```python
from build123d import *

# Parameters (mm, degrees)
SKETCH1_W           = 58.42
SKETCH1_H           = 58.42
SKETCH1_R           = 2.1
SKETCH1_R_2         = 5.5
SKETCH1_R_3         = 2.05
BOSS_EXTRUDE1_DEPTH = 6.35
CHAMFER1_SIZE       = 2.48
CHAMFER2_SIZE       = 3.1


with BuildPart() as part:
    # Sketch1 → Boss-Extrude1 (new body)
    with BuildSketch(Plane(origin=(0, 0, 0), x_dir=(1, 0, 0), z_dir=(0, 1, 0))):
        with Locations((29.21, 29.21)):
            Rectangle(SKETCH1_W, SKETCH1_H)
        with Locations(Location((5.64, 52.78, 0), (0, 0, 270))):
            Circle(SKETCH1_R, mode=Mode.SUBTRACT)
        with Locations(Location((52.78, 52.78, 0), (0, 0, 270))):
            Circle(SKETCH1_R, mode=Mode.SUBTRACT)
        with Locations(Location((52.78, 5.64, 0), (0, 0, 270))):
            Circle(SKETCH1_R, mode=Mode.SUBTRACT)
        with Locations(Location((5.64, 5.64, 0), (0, 0, 270))):
            Circle(SKETCH1_R, mode=Mode.SUBTRACT)
        with Locations(Location((29.21, 29.21, 0), (0, 0, 270))):
            Circle(SKETCH1_R_2, mode=Mode.SUBTRACT)
        with Locations(Location((13.653650814, 44.766349186, 0), (0, 0, 270))):
            Circle(SKETCH1_R_3, mode=Mode.SUBTRACT)
        with Locations(Location((44.766349186, 44.766349186, 0), (0, 0, 270))):
            Circle(SKETCH1_R_3, mode=Mode.SUBTRACT)
        with Locations(Location((44.766349186, 13.653650814, 0), (0, 0, 270))):
            Circle(SKETCH1_R_3, mode=Mode.SUBTRACT)
        with Locations(Location((13.653650814, 13.653650814, 0), (0, 0, 270))):
            Circle(SKETCH1_R_3, mode=Mode.SUBTRACT)
    extrude(amount=BOSS_EXTRUDE1_DEPTH)

    # Chamfer1
    chamfer1_edges = [part.edges().sort_by_distance(p)[0] for p in [
        (13.653650814, 0, -46.816349186),
        (44.766349186, 0, -46.816349186),
        (44.766349186, 0, -15.703650814),
        (13.653650814, 0, -15.703650814),
    ]]
    chamfer(chamfer1_edges, length=CHAMFER1_SIZE)

    # Chamfer2
    chamfer2_edges = [part.edges().sort_by_distance(p)[0] for p in [
        (5.64, 6.35, -54.88),
        (52.78, 6.35, -54.88),
        (52.78, 6.35, -7.74),
        (5.64, 6.35, -7.74),
    ]]
    chamfer(chamfer2_edges, length=CHAMFER2_SIZE)


solid = part.part
```
Input: part model. Units: mm. Frame: model coordinates. Round coordinates to 2 decimals unless told otherwise and drop trailing zeros. Order: outer loops, then holes, each group sorted by start corner. A loop starts at its lowest first (then second) coordinate and runs counter-clockwise, first axis right, second up. Notation, with made-up numbers: (50.5, 62) - (94.5, 62) arc R8 ccw to (94.5, 74) - close; hole circle Ø11 at (68, 5.25). An arc over 180 degrees is marked (long way). One line per question, with ' | ' between items. Start each with the question number.
1) Cut plane C-C, the plane x = 29.21. Return the cut outline in (y, z).
2) Cut plane A-A, the plane x = 52.78. Return the cut outline in (y, z), then the cut area to 3 significant figures.
3) Pull-direction query (Z, two-part tool) for faces 1 (the flat face through (22, 6.35, -30)), 2 (the conical face through (6.316, 3.401, -3.493)), 3 (the flat face through (29, 3, -58.42)); classes: +Z half, -Z half, draft (parallel to the pull), parting line (faces both ways), or undercut.
4) Contact query for flat-ended pins moving along their axis: P1, Ø4.5, axis at x = 13.65, z = -44.77, coming from the -Y side; P2, Ø4, axis at x = 52.78, z = -5.64, coming from the -Y side; P3, Ø5.5, axis at x = 5.64, z = -52.78, coming from the +Y side; P4, Ø6.5, axis at x = 5.64, z = -5.64, coming from the +Y side. Output: stop coordinate, or through.
5) Cut plane D-D, the plane y = 4. Give the number of separate pieces and of enclosed holes in the cut face, then the cut area to 3 significant figures.
6) Cut plane B-B, the plane z = -5.64. Return the cut outline in (x, y), then the cut area to 3 significant figures.
7) Ray query, probe 1 along X at (y, z) = (1.15, -52.78); probe 2 along Z at (x, y) = (14, 4.5); probe 3 along X at (y, z) = (5.75, -46). Return the intervals inside material, ascending.
Worked out:
1) outline: (0, -58.42) - (6.35, -58.42) - (6.35, -34.71) - (0, -34.71) - close; (0, -23.71) - (6.35, -23.71) - (6.35, 0) - (0, 0) - close
2) outline: (0, -58.42) - (6.35, -58.42) - (6.35, -57.98) - (3.25, -54.88) - (0, -54.88) - close; (0, -50.68) - (3.25, -50.68) - (6.35, -47.58) - (6.35, -10.84) - (3.25, -7.74) - (0, -7.74) - close; (0, -3.54) - (3.25, -3.54) - (6.35, -0.44) - (6.35, 0) - (0, 0) - close | area: 298 mm^2
3) face 1: draft | face 2: undercut | face 3: -Z half
4) P1: stops at y = 2.27 | P2: passes through | P3: stops at y = 3.9 | P4: stops at y = 4.4
5) separate pieces: 1 | enclosed holes: 9 | area: 3,160 mm^2
6) outline: (0, 0) - (3.54, 0) - (3.54, 3.25) - (0.44, 6.35) - (0, 6.35) - close; (7.74, 0) - (50.68, 0) - (50.68, 3.25) - (47.58, 6.35) - (10.84, 6.35) - (7.74, 3.25) - close; (54.88, 0) - (58.42, 0) - (58.42, 6.35) - (57.98, 6.35) - (54.88, 3.25) - close | area: 298 mm^2
7) probe 1: x = 0 to 3.54, 7.74 to 50.68, 54.88 to 58.42 | probe 2: z = -58.42 to -46.79, -42.75 to -15.67, -11.63 to 0 | probe 3: x = 0 to 12.02, 15.29 to 43.13, 46.4 to 58.42
